Answer from the drawing. Dimensions are ordinates in mm from the lowest x, y and z of the part. A direction names the side the tool comes from. Coordinates: 2 decimals unless noted, no trailing zeros. Order: outer loops, then holes, each group sorted by start corner. A loop starts at its lowest first (then second) coordinate and runs counter-clockwise, first axis right, second up. Notation, with made-up numbers: M 2.5,10.5 L 61.5,10.5 A24 ccw 61.5,46.5 Z; hole C -3.75,-28 d2. An arc over 180 degrees is marked long. Use a Markdown table: item, result.
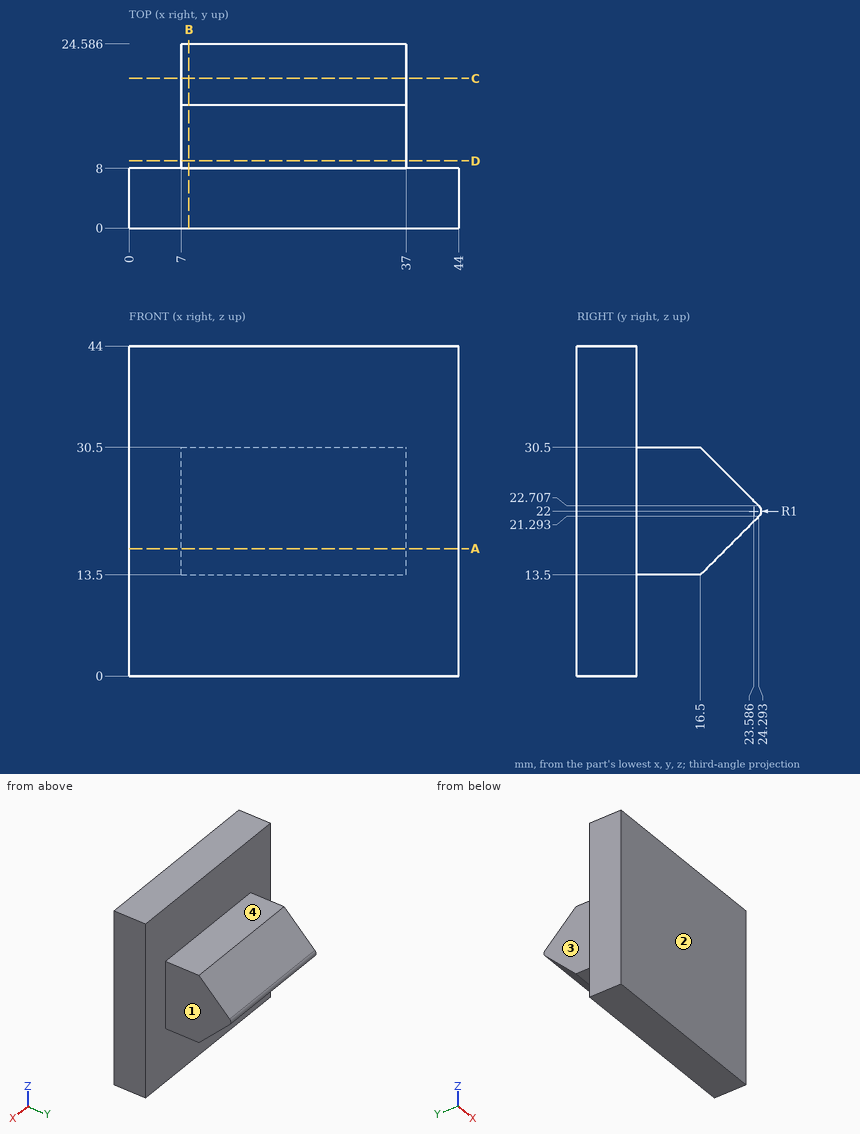
(1) A cutting plane is placed at D-D (y = 9). Determine the outline of the cut face in (x, z), then the cut area to 3 significant figures.
Conclusion:
| item | result |
|---|---|
| outline | M 7,13.5 L 37,13.5 L 37,30.5 L 7,30.5 Z |
| area | 510 mm2 |
(2) A cutting plane is placed at B-B (x = 8). Determine the outline of the cut face in (y, z).
Conclusion:
| item | result |
|---|---|
| outline | M 0,0 L 8,0 L 8,13.5 L 16.5,13.5 L 24.29,21.29 A1 ccw 24.29,22.71 L 16.5,30.5 L 8,30.5 L 8,44 L 0,44 Z |
(3) A cutting plane is placed at C-C (y = 20). Determine the outline of the cut face in (x, z).
Conclusion:
| item | result |
|---|---|
| outline | M 7,17 L 37,17 L 37,27 L 7,27 Z |
(4) Given P1, Ø13.5, axis at y = 17.5, z = 18, coming from the +X side; P2, Ø1, axis at x = 12, y = 13.5, coming from the -Z side; P3, Ø1.5, axis at y = 14.5, z = 13, coming from the -X side, each flat-ended and moving along its own axis, determine where each tip first touches the part or whether it passes through.
Conclusion:
| item | result |
|---|---|
| P1 | x = 37 |
| P2 | z = 13.5 |
| P3 | x = 7 |
(5) A cutting plane is placed at A-A (z = 17). Determine the outline of the cut face in (x, y), then the cut area to 3 significant figures.
Conclusion:
| item | result |
|---|---|
| outline | M 0,0 L 44,0 L 44,8 L 37,8 L 37,20 L 7,20 L 7,8 L 0,8 Z |
| area | 712 mm2 |
(6) Which of the six approach directions +Z, -Z, +X, -X, +Y, -Y give full straight-line access (tool end or side, diameter ignored) to the marked faces 1, 2, 3 and 4?
Conclusion:
| item | result |
|---|---|
| face 1 | +Z, -Z, +X, +Y |
| face 2 | +Z, -Z, +X, -X, -Y |
| face 3 | +Z, -Z, -X, +Y |
| face 4 | +Z, +X, -X, +Y |
(7) Straight lines are drawn through the part: L1, parallel to X at y = 15.5, z = 30; L2, parallel to Y at x = 3.5, z = 28.5; L3, parallel to Z at x = 34, y = 15. For each, find the intervals that lie inside material, in ascending order.
Conclusion:
| item | result |
|---|---|
| L1 | 7 to 37 |
| L2 | 0 to 8 |
| L3 | 13.5 to 30.5 |
